from build123d import *

# Parameters (mm, degrees)
BOSS_EXTRUDE1_DEPTH          = 60
SKETCH2_R                    = 1.5
CUT_EXTRUDE2_DEPTH           = 7.35
CSK_FOR_M3_SFHCS1_AT_2_COUNT = 2
CSK_FOR_M3_SFHCS1_AT_2_PITCH = 34.6
CHAMFER1_SIZE                = 0.762


with BuildPart() as part:
    # Sketch1 → Boss-Extrude1 (new body)
    with BuildSketch(Plane(origin=(0, 0, 0), x_dir=(1, 0, 0), z_dir=(0, 1, 0))):
        Polygon((-3.175, 6.35), (3.175, 6.35), (3.175, 3.175), (12.7, 3.175), (12.7, 0), (-12.7, 0), (-12.7, 3.175), (-3.175, 3.175), align=None)
    extrude(amount=BOSS_EXTRUDE1_DEPTH)

    # Sketch2 → Cut-Extrude2 (cut, through all)
    with BuildSketch(Plane(origin=(0, 0, -6.35), x_dir=(-1, 0, 0), z_dir=(0, 0, -1))):
        with Locations((0, 47.3)):
            Circle(SKETCH2_R)
        with Locations((0, 12.7)):
            Circle(SKETCH2_R)
    extrude(amount=-CUT_EXTRUDE2_DEPTH, mode=Mode.SUBTRACT)

    # Sketch4 → CSK for M3 SFHCS1 (revolve, cut)
    with BuildSketch(Plane(origin=(0, 12.7, -6.35), x_dir=(0, 1, 0), z_dir=(1, 0, 0))):
        Polygon((0, 0), (0, 6.35), (1.8, 6.35), (1.8, 2.83), (3.36, 1.27), (3.36, 0), align=None)
    csk_for_m3_sfhcs1 = revolve(axis=Axis((0, 12.7, -12.7), (0, 0, 1)), mode=Mode.SUBTRACT)

    # CSK for M3 SFHCS1 at 2: CSK for M3 SFHCS1 ×2
    with Locations(*[(0, i * CSK_FOR_M3_SFHCS1_AT_2_PITCH, 0) for i in range(1, CSK_FOR_M3_SFHCS1_AT_2_COUNT)]):
        add(csk_for_m3_sfhcs1, mode=Mode.SUBTRACT)

    # Chamfer1
    chamfer1_edges = [part.edges().sort_by_distance(p)[0] for p in [
        (12.7, 30, -3.175),
        (-12.7, 30, -3.175),
    ]]
    chamfer(chamfer1_edges, length=CHAMFER1_SIZE)


solid = part.part
The model under review builds one solid part; all positions refer to its coordinate system, in mm. A direction names the side the tool comes from. Round coordinates to 2 decimals unless told otherwise and drop trailing zeros. Loops run counter-clockwise (first coordinate to the right, second up) from the corner with the lowest first, then second, coordinate; pieces in that order, holes last. Notation, with made-up numbers: M 36.25,-13.75 L 76.25,-13.75 A10 cw 76.25,3.25 Z; hole C 23.5,-3.5 d6. An arc over 180 degrees is marked long. Answer as CSV lines item,"result". Start each with the question number.
Item 1: Consider section C-C (x = -6.75). Write out the cut boundary in (y, z) (3 decimals).
Item 2: Wall thickness on line 1 (Y direction, x = 0, z = -2.45); line 2 (X direction, y = 12.7, z = -1.5); line 3 (X direction, y = 56, z = -4.25) (3 decimals): over which ranges is each line inside the solid? List them lowest first. Write a range as [from, to].
Item 3: For faces 1 (the face through (-8, 30, -3.175)), 2 (the face through (3.175, 30, -5)), 3 (the face through (0, 4, -6.35)), 4 (the face through (0, 0, -3)), 5 (the face through (-0.06, 43.94, -5.72)), list the 3-axis set-ups (+Z, -Z, +X, -X, +Y, -Y) from which the entire face can be reached by the end or side of a thin tool; tool diameter is ignored.
Item 4: Consider section B-B (x = 0). Write out the cut boundary in (y, z), then the cut area to 3 significant figures.
Item 5: Insertion check: P1, Ø3.5, axis at y = 33.5, z = -4.5, coming from the +X side; P2, Ø4, axis at x = -7.5, y = 13.5, coming from the -Z side (3 decimals); P3, Ø1.6, axis at y = 15, z = -5, coming from the -X side (3 decimals). Each pin has a flat end and moves straight along its axis. Give the tip position at first contact, or say it passes through.
Item 6: Consider section A-A (y = 47.3). Write out the cut boundary in (x, z) (3 decimals), then the cut area to 3 significant figures.
Answer:
1,outline,"M 0,-3.175 L 60,-3.175 L 60,0 L 0,0 Z"
2,line 1,"y = [0, 10.9], [14.5, 45.5], [49.1, 60]"
2,line 2,"x = [-12.7, -1.8], [1.8, 12.7]"
2,line 3,"x = [-3.175, 3.175]"
3,face 1,"-Z, -X, +Y, -Y"
3,face 2,"-Z, +X, +Y, -Y"
3,face 3,"-Z, +X, -X, +Y, -Y"
3,face 4,"+Z, -Z, +X, -X, -Y"
3,face 5,"-Z"
4,outline,"M 0,-6.35 L 9.34,-6.35 L 9.34,-5.08 L 10.9,-3.52 L 10.9,0 L 0,0 Z; M 14.5,-3.52 L 16.06,-5.08 L 16.06,-6.35 L 43.94,-6.35 L 43.94,-5.08 L 45.5,-3.52 L 45.5,0 L 14.5,0 Z; M 49.1,-3.52 L 50.66,-5.08 L 50.66,-6.35 L 60,-6.35 L 60,0 L 49.1,0 Z"
4,area,"322 mm^2"
5,P1,"stops at x = 12.36"
5,P2,"stops at z = -3.175"
5,P3,"stops at x = -3.175"
6,outline,"M -12.7,-2.413 L -11.938,-3.175 L -3.175,-3.175 L -3.175,-4.895 L -1.8,-3.52 L -1.8,0 L -12.7,0 Z; M 1.8,-3.52 L 3.175,-4.895 L 3.175,-3.175 L 11.938,-3.175 L 12.7,-2.413 L 12.7,0 L 1.8,0 Z"
6,area,"71.5 mm^2"
